Autodesk Inventor part; units mm, degrees
ref_plane "YZ Plane" through (0, 0, 0) normal (1, 0, 0) x (0, 1, 0)
ref_plane "XZ Plane" through (0, 0, 0) normal (0, 1, 0) x (-1, 0, 0)
ref_plane "XY Plane" through (0, 0, 0) normal (0, 0, 1) x (1, 0, 0)
sketch "Sketch1" plane through (0, 0, 0) normal (0, 0, 1) x (1, 0, 0)
  line L0 (0, 18) -> (43.25, 18)
  line L1 (43.25, 18) -> (43.25, 0)
  line L2 (43.25, 0) -> (0, 0)
  line L3 (0, 0) -> (0, 9)
  line L4 (0, 12.81) -> (5.08, 12.81)
  line L5 (5.08, 12.81) -> (5.08, 5.19)
  line L6 (5.08, 5.19) -> (0, 5.19)
  line L7 (0, 5.19) -> (0, 9)
  line L8 (0, 9) -> (43.25, 9) construction
  line L9 (0, 9) -> (0, 18)
  line L10 (0, 9) -> (0, 12.81)
  dimension "d0" = 43.25
  dimension "d1" = 18
  dimension "d3" = 7.62
  dimension "d4" = 5.08
extrude "Extrusion1" add sketch "Sketch1" along normal blind 2 contours L0 L1 L2 L3 L6 L5 L4 L9
extrude "Extrusion2" add sketch "Sketch1" along normal blind 3 and the other way blind 8.25 contours L4 L5 L6 L3 L9
sketch "Sketch2" plane through (43.25, 0, 0) normal (1, 0, 0) x (0, 0, -1)
  line L0 (0, 12) -> (1.25, 12)
  line L1 (1.25, 6) -> (0, 6)
  line L2 (0, 6) -> (0, 9)
  line L3 (3.25, 5.5) -> (1.25, 5.5)
  line L4 (1.25, 5.5) -> (1.25, 6)
  line L5 (1.25, 12.5) -> (3.25, 12.5)
  line L6 (3.25, 12.5) -> (3.25, 5.5)
  line L7 (0, 9) -> (3.25, 9) construction
  line L8 (0, 9) -> (0, 12)
  line L9 (1.25, 9) -> (1.25, 12) construction
  line L10 (1.25, 12) -> (1.25, 12.5)
  line L11 (1.25, 6) -> (1.25, 9) construction
  line L12 (0, 18) -> (0, 0)
  line L13 (0, 0) -> (0, 18)
  point P0 (0, 12.81)
  point P1 (0, 5.19)
  point P2 (0, 9)
  point P3 (0, 9)
  dimension "d9" = 6
  dimension "d10" = 1.25
  dimension "d12" = 7
  dimension "d13" = 2
extrude "Extrusion3" add sketch "Sketch2" along normal blind 1.25 and the other way blind 8
sketch "Sketch3" plane through (0, 0, 2) normal (0, 0, 1) x (1, 0, 0)
  line L0 (2.625, 18) -> (40.625, 18)
  line L1 (40.625, 18) -> (40.625, 16)
  line L2 (40.625, 16) -> (2.625, 16)
  line L3 (2.625, 16) -> (2.625, 18)
  line L4 (0, 18) -> (0, 12.81)
  line L5 (2.625, 17) -> (0, 18) construction
  line L6 (40.625, 17) -> (43.25, 18) construction
  line L7 (43.25, 0) -> (43.25, 18)
  line L8 (43.25, 9) -> (0, 9) construction
  line L9 (0, 5.19) -> (0, 12.81)
  line L10 (2.625, 0) -> (40.625, 0)
  line L11 (40.625, 0) -> (40.625, 2)
  line L12 (40.625, 2) -> (2.625, 2)
  line L13 (2.625, 2) -> (2.625, 0)
  point P0 (0, 0)
  dimension "d20" = 38
  dimension "d21" = 2
extrude "Extrusion4" add sketch "Sketch3" along normal blind 8.25 and the other way blind 3
properties part number "NANO"
Verification items for the finished model (mm, model axes). A direction names the side the tool comes from. Give positions to 0.01 mm unless a question says otherwise; leave off trailing zeros. Order: outer loops, then holes, each group sorted by start corner. A loop starts at its lowest first (then second) coordinate and runs counter-clockwise, first axis right, second up. Notation, with made-up numbers: (22.5, -9.75) -> (74.5, -9.75) arc R26 ccw to (74.5, 12.25) -> close; hole circle Ø6 at (78, 45.5). An arc over 180 degrees is marked (long way). Answer as CSV lines item,"result".
Q1. Sectioned sample at D-D on z = -4. Record the cut outline in (x, y).
Solutions:
outline,"(0, 5.19) -> (5.08, 5.19) -> (5.08, 12.81) -> (0, 12.81) -> close"
Q2. Scan lines: probe 1 along Z at (x, y) = (28.5, 14.75); probe 2 along X at (y, z) = (16.25, 5.75) (3 decimals); probe 3 along Z at (x, y) = (15, 1.5). Record each from-to range of solid material in increasing order.
Solutions:
probe 1,"z = 0 to 2"
probe 2,"x = 2.625 to 40.625"
probe 3,"z = -1 to 10.25"
Q3. Sectioned sample at C-C on x = 41.5. Record the cut outline in (y, z).
Solutions:
outline,"(0, 0) -> (6, 0) -> (6, -1.25) -> (5.5, -1.25) -> (5.5, -3.25) -> (12.5, -3.25) -> (12.5, -1.25) -> (12, -1.25) -> (12, 0) -> (18, 0) -> (18, 2) -> (0, 2) -> close"
Q4. Sectioned sample at A-A on z = 2.5. Record the cut outline in (x, y) (3 decimals).
Solutions:
outline,"(0, 5.19) -> (5.08, 5.19) -> (5.08, 12.81) -> (0, 12.81) -> close; (2.625, 0) -> (40.625, 0) -> (40.625, 2) -> (2.625, 2) -> close; (2.625, 16) -> (40.625, 16) -> (40.625, 18) -> (2.625, 18) -> close"
Q5. Sectioned sample at B-B on y = 17. Record the cut outline in (x, z) (3 decimals).
Solutions:
outline,"(0, 0) -> (2.625, 0) -> (2.625, -1) -> (40.625, -1) -> (40.625, 0) -> (43.25, 0) -> (43.25, 2) -> (40.625, 2) -> (40.625, 10.25) -> (2.625, 10.25) -> (2.625, 2) -> (0, 2) -> close"
Q6. Release check for a two-part mould opening along Y. For faces 1 (the flat face through (21, 1, 10.25)), 2 (the flat face through (40, 12.5, -2)), 3 (the flat face through (21.9, 2, -0.5)) record: +Y half, -Y half, draft (parallel to the pull), parting line (faces both ways), or undercut.
Solutions:
face 1,"draft"
face 2,"+Y half"
face 3,"undercut"
Q7. Depth check by flat-ended pin: pin 1 (2 mm diameter, centred on y = 1, z = 4.5, fed in from -X) (3 decimals); pin 2 (1 mm diameter, centred on y = 16.5, z = 7.5, fed in from +X) (3 decimals); pin 3 (6 mm diameter, centred on y = 2, z = 2, fed in from +X); pin 4 (4 mm diameter, centred on y = 9, z = 5.5, fed in from -X). Enter the tip coordinate at first touch or a pass-through.
Solutions:
pin 1,"stops at x = 2.625"
pin 2,"stops at x = 40.625"
pin 3,"stops at x = 43.25"
pin 4,"passes through"
Q8. Access from +Z, -Z, +X, -X, +Y, -Y to the whole of each face (thin tool, end or side, straight path). Record for faces 4 (the flat face through (43.25, 9, 1)), 5 (the flat face through (21, 17, -1)), 6 (the flat face through (35.25, 9, -2)), 7 (the flat face through (22, 16, 6)).
Solutions:
face 4,"+Z, +X, +Y, -Y"
face 5,"-Z, +X, -X, +Y"
face 6,"-Z"
face 7,"+Z, +X, -X"
